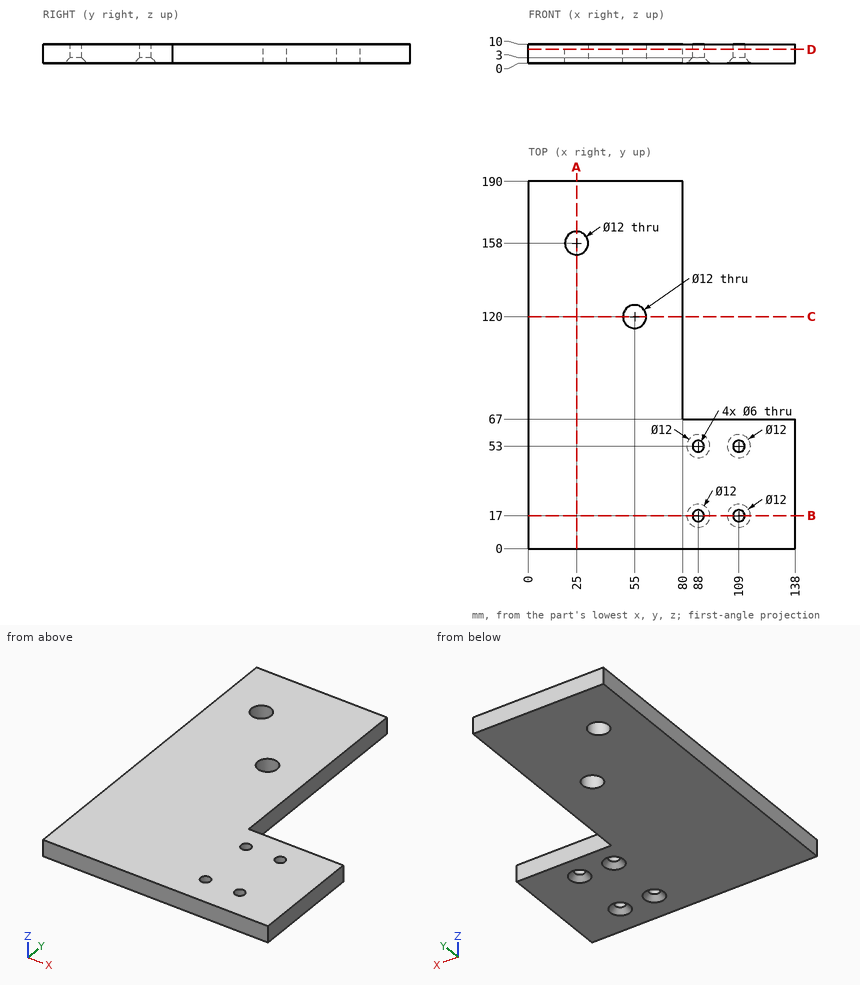
Source: three-view drawing plus pictorial views. Frame: mm from the lowest corner of the part. Coordinates: 2 decimals unless noted, no trailing zeros. Loops run counter-clockwise (first coordinate to the right, second up) from the corner with the lowest first, then second, coordinate; pieces in that order, holes last. Notation, with made-up numbers: (54.25, 28.5) - (100.25, 28.5) arc R23 cw to (100.25, 48.5) - close; hole circle Ø6 at (51.25, 11). An arc over 180 degrees is marked (long way). One line per question, with ' | ' between items.
1) First-contact query: P1, Ø5, axis at y = 109, z = 6, coming from the +X side; P2, Ø3.5, axis at x = 109, y = 53, coming from the -Z side. Flat tips, straight axial feed; report the tip coordinate or a pass-through.
Report:
P1: stops at x = 80 | P2: passes through
2) Section C-C, the plane y = 120. Return loops of the section in (x, z), then the cut area to 3 significant figures.
Report:
outline: (0, 0) - (49, 0) - (49, 10) - (0, 10) - close; (61, 0) - (80, 0) - (80, 10) - (61, 10) - close | area: 680 mm²
3) Section D-D, the plane z = 7.25. Return loops of the section in (x, y), then the cut area to 3 significant figures.
Report:
outline: (0, 0) - (138, 0) - (138, 67) - (80, 67) - (80, 190) - (0, 190) - close; hole circle Ø12 at (25, 158); hole circle Ø12 at (55, 120); hole circle Ø6 at (88, 17); hole circle Ø6 at (88, 53); hole circle Ø6 at (109, 17); hole circle Ø6 at (109, 53) | area: 18,700 mm²
4) Section B-B, the plane y = 17. Return loops of the section in (x, z).
Report:
outline: (0, 0) - (82, 0) - (85, 3) - (85, 10) - (0, 10) - close; (91, 3) - (94, 0) - (103, 0) - (106, 3) - (106, 10) - (91, 10) - close; (112, 3) - (115, 0) - (138, 0) - (138, 10) - (112, 10) - close
5) Line query: line 1 along Y through (x, z) = (109, 5); line 2 along Y through (x, z) = (25, 2.75); line 3 along Y through (x, z) = (55, 5.75). Output: solid intervals per line, ascending.
Report:
line 1: y = 0 to 14, 20 to 50, 56 to 67 | line 2: y = 0 to 152, 164 to 190 | line 3: y = 0 to 114, 126 to 190
6) Section A-A, the plane x = 25. Return loops of the section in (y, z).
Report:
outline: (0, 0) - (152, 0) - (152, 10) - (0, 10) - close; (164, 0) - (190, 0) - (190, 10) - (164, 10) - close
